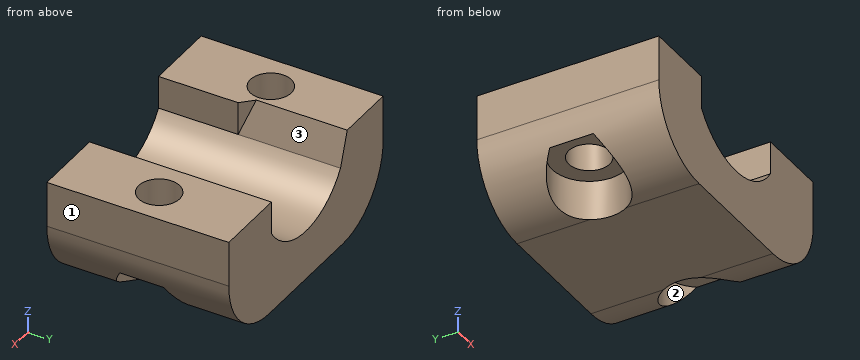
Solid Edge part; units mm, degrees
sketch "Sketch1" plane through (0, 0, 0) normal (1, 0, 0) x (0, 1, 0)
  line L0 (-8, 5) -> (8, 5)
  line L1 (8, 5) -> (8, -5)
  line L2 (8, -5) -> (-8, -5)
  line L3 (-8, -5) -> (-8, 5)
  dimension "D1" = 8
  dimension "D2" = 8
extrude "Protrusion1" add sketch "Sketch1" along normal mid plane 23
sketch "Sketch2" plane through (0, 8, 0) normal (0, 1, 0) x (0, 0, -1)
  line L0 (-5, 5.15) -> (-5, -5.15)
  line L1 (-5, -5.15) -> (-2.1, -5.15)
  arc A0 (-2.1, -5.15) -> (-2.1, 5.15) centre (-5.5522, 0) ccw
  line L2 (-5, 5.15) -> (-2.1, 5.15)
  dimension "D1" = 5
extrude "Extrusionsausschnitt_1" cut sketch "Sketch2" against normal blind 22.6589
fillet "Verrundung_1" radius 6 2 edges at (-11.5, 0, -5) (11.5, 0, -5)
hole "Bohrung_1" at (-8.325, 0, -5) direction (0, 0, 1) diameter 3.6 end through all counterbore diameter 6.5 counterbore depth 3.5
hole "Hole1" at (8.325, 0, -5) direction (0, 0, 1) diameter 3.6 end through all counterbore diameter 6.5 counterbore depth 3.5
sketch "Sketch3" plane through (0, 8, 0) normal (0, 1, 0) x (-1, 0, 0)
  line L0 (5.15, 2.1) -> (6.15, 5)
  line L1 (6.15, 5) -> (5.15, 5)
  line L2 (5.15, 5) -> (5.15, 2.1)
  dimension "D1" = 6.15
extrude "Extrusionsausschnitt_2" cut sketch "Sketch3" against normal blind 8
chamfer "Fase_1" distance 1 angle 45 1 edges at (-5.15, 0, 3.55)
Geometry check sheet. Reference: the model listing, model coordinates, mm. Face numbers are marked on the shaded views. A direction names the side the tool comes from. Round coordinates to 2 decimals unless told otherwise and drop trailing zeros. Loops run counter-clockwise (first coordinate to the right, second up) from the corner with the lowest first, then second, coordinate; pieces in that order, holes last. Notation, with made-up numbers: (41.5, -29) -> (94.5, -29) arc R30 ccw to (94.5, -6) -> close; hole circle Ø6 at (-14.5, 27). An arc over 180 degrees is marked (long way). Use a Markdown table: item, result.
(1) Set-up check for the marked faces 1, 2 and 3: record each of +Z, -Z, +X, -X, +Y, -Y from which the full face is reachable in a straight line by a thin tool's end or side.
Calculated:
| item | result |
|---|---|
| face 1 | +Z, -Z, +X, +Y, -Y |
| face 2 | -Z |
| face 3 | +Z, +Y |
(2) Sectioned sample at A-A (y = -0.75). Enter the section's corners in (x, z), then the cut area to 3 significant figures.
Calculated:
| item | result |
|---|---|
| outline | (-11.5, 1) arc R6 ccw to (-10.95, -1.5) -> (-9.96, -1.5) -> (-9.96, 5) -> (-11.5, 5) -> close; (-6.69, -1.5) -> (-5.16, -1.5) -> (-5.16, -5) -> (5.16, -5) -> (5.16, -1.5) -> (6.69, -1.5) -> (6.69, 5) -> (5.15, 5) -> (5.15, 2.1) arc R6.2 cw to (-5.15, 2.1) -> (-5.4, 2.82) -> (-5.4, 5) -> (-6.69, 5) -> close; (9.96, -1.5) -> (10.95, -1.5) arc R6 ccw to (11.5, 1) -> (11.5, 5) -> (9.96, 5) -> close |
| area | 91.8 mm² |
(3) Sectioned sample at C-C (y = 6). Enter the section's corners in (x, z), then the cut area to 3 significant figures.
Calculated:
| item | result |
|---|---|
| outline | (-11.5, 1) arc R6 ccw to (-5.5, -5) -> (5.5, -5) arc R6 ccw to (11.5, 1) -> (11.5, 5) -> (5.15, 5) -> (5.15, 2.1) arc R6.2 cw to (-5.15, 2.1) -> (-6.15, 5) -> (-11.5, 5) -> close |
| area | 163 mm² |
(4) Sectioned sample at D-D (z = -3.25). Enter the section's corners in (x, y) (3 decimals), then the cut area to 3 significant figures.
Calculated:
| item | result |
|---|---|
| outline | (-9.735, -8) -> (9.735, -8) -> (9.735, -2.928) arc R3.25 cw (long way) to (9.735, 2.928) -> (9.735, 8) -> (-9.735, 8) -> (-9.735, 2.928) arc R3.25 cw (long way) to (-9.735, -2.928) -> close |
| area | 261 mm² |
(5) Go/stop test with flat-tipped pins: P1, Ø3, axis at x = -8.325, y = 0, coming from the -Z side; P2, Ø1.5, axis at y = 6, z = -1, coming from the +X side; P3, Ø3, axis at x = 7.5, y = -1, coming from the -Z side. Record where each tip stops, or that it passes through.
Calculated:
| item | result |
|---|---|
| P1 | through |
| P2 | x = 11.37 |
| P3 | z = -1.5 |
(6) Sectioned sample at B-B (z = 1.5). Enter the section's corners in (x, y) (3 decimals), then the cut area to 3 significant figures.
Calculated:
| item | result |
|---|---|
| outline | (-11.5, -8) -> (-4.693, -8) -> (-4.693, 8) -> (-11.5, 8) -> close; (4.693, -8) -> (11.5, -8) -> (11.5, 8) -> (4.693, 8) -> close; hole circle Ø3.6 at (-8.325, 0); hole circle Ø3.6 at (8.325, 0) |
| area | 197 mm² |
(7) Scan lines: probe 1 along X at (y, z) = (-6.5, 3.25); probe 2 along X at (y, z) = (0, 3.5) (3 decimals); probe 3 along X at (y, z) = (-1.25, 4.5). Record each from-to range of solid material in increasing order.
Calculated:
| item | result |
|---|---|
| probe 1 | -11.5 to -5.15, 5.15 to 11.5 |
| probe 2 | -11.5 to -10.125, -6.525 to -5.633, 5.15 to 6.525, 10.125 to 11.5 |
| probe 3 | -11.5 to -9.62, -7.03 to -5.15, 5.15 to 7.03, 9.62 to 11.5 |
